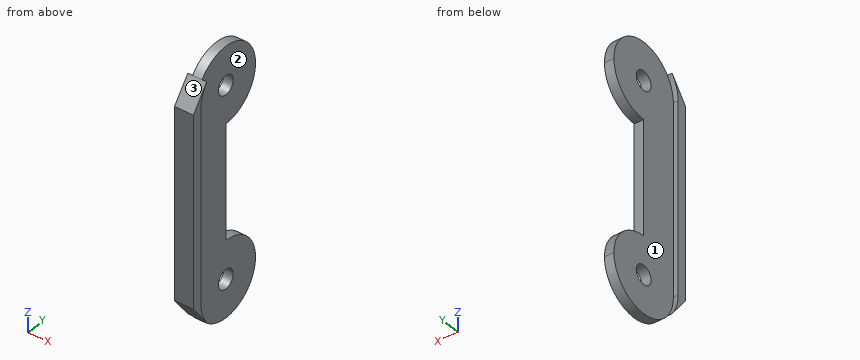
```python
from build123d import *

# Parameters (mm, degrees)
F1_DEPTH = 2.5
F0_R     = 2.5
F2_DEPTH = 1.25


with BuildPart() as f1:
    # F0 (on Right) → F1 (new body, symmetric)
    with BuildSketch(Plane.YZ):
        with BuildLine():
            ThreePointArc((-10, 25), (-9.486833, 28.162278), (-8, 31))
            Line((-8, 31), (-12.5, 25))
            Line((-12.5, 25), (-12.5, -25))
            Line((-12.5, -25), (-8, -31))
            ThreePointArc((-8, -31), (-9.486833, -28.162278), (-10, -25))
            Line((-10, -25), (-10, 25))
        make_face()
    extrude(amount=F1_DEPTH, both=True)

    # F0 (on Right) → F2 (join, symmetric)
    with BuildSketch(Plane.YZ):
        with BuildLine():
            ThreePointArc((0, 15), (7.071068, 17.928932), (10, 25))
            ThreePointArc((10, 25), (3.162278, 34.486833), (-8, 31))
            ThreePointArc((-8, 31), (-9.486833, 28.162278), (-10, 25))
            ThreePointArc((-10, 25), (-7.071068, 17.928932), (0, 15))
        make_face()
        with Locations((0, 25)):
            Circle(F0_R, mode=Mode.SUBTRACT)
        with BuildLine():
            Line((0, -15), (0, 15))
            ThreePointArc((0, 15), (-7.071068, 17.928932), (-10, 25))
            Line((-10, 25), (-10, -25))
            ThreePointArc((-10, -25), (-7.071068, -17.928932), (0, -15))
        make_face()
        with BuildLine():
            ThreePointArc((10, -25), (7.071068, -17.928932), (0, -15))
            ThreePointArc((0, -15), (-7.071068, -17.928932), (-10, -25))
            ThreePointArc((-10, -25), (-9.486833, -28.162278), (-8, -31))
            ThreePointArc((-8, -31), (3.162278, -34.486833), (10, -25))
        make_face()
        with Locations((0, -25)):
            Circle(F0_R, mode=Mode.SUBTRACT)
    extrude(amount=F2_DEPTH, both=True)


solid = f1.part
```
Could you check a few things on this model? Use its own coordinates, in mm. Face numbers are marked on the shaded views. A direction names the side the tool comes from. Coordinates: 2 decimals unless noted, no trailing zeros. Write each loop counter-clockwise with the first axis right and the second up, starting at its lowest first coordinate (ties: lowest second). Pieces come first, ordered by that corner, then holes. Notation, with made-up numbers: (20, 37) -> (36, 37) arc R26 ccw to (36, 65) -> close; hole circle Ø5 at (61.5, 56). An arc over 180 degrees is marked (long way). One line per question, with ' | ' between items. Start each with the question number.
1. If we section it at A-A (y = 8): Please give me the cut outline in (x, z), and give its area (3 significant figures).
2. Will these pins go through, and if not, where does the flat tip stop? P1, Ø1.4, axis at x = 1.5, z = -6, coming from the +Y side; P2, Ø8, axis at y = 0, z = -25, coming from the +X side; P3, Ø2, axis at x = -1, y = 5, coming from the -Z side.
3. If we section it at B-B (x = 0.05): Please give me the cut outline in (y, z).
4. For the marked faces 1, 2 and 3, which set-ups out of +Z, -Z, +X, -X, +Y, -Y let a thin tool reach every point of the face, with its end or its side?
5. If we section it at C-C (z = -13): Please give me the cut outline in (x, y), and give its area (3 significant figures).
6. If we section it at D-D (z = 26): Please give me the cut outline in (x, y).
7. Please list where these lines run through material, in increasing order: line 1 along X through (y, z) = (-5, -5.5); line 2 along Y through (x, z) = (0.1, 6); line 3 along Z through (x, y) = (0.45, 5.5).
Return value:
1) outline: (-1.25, -31) -> (1.25, -31) -> (1.25, -19) -> (-1.25, -19) -> close; (-1.25, 19) -> (1.25, 19) -> (1.25, 31) -> (-1.25, 31) -> close | area: 60.0 mm²
2) P1: stops at y = 0 | P2: stops at x = 1.25 | P3: stops at z = -34.17
3) outline: (-12.5, -25) -> (-8, -31) arc R10 ccw (long way) to (0, -15) -> (0, 15) arc R10 ccw (long way) to (-8, 31) -> (-12.5, 25) -> close; hole circle Ø5 at (0, -25); hole circle Ø5 at (0, 25)
4) face 1: -X, +Y | face 2: +X, +Y | face 3: +Z, +X, -X, -Y
5) outline: (-2.5, -12.5) -> (2.5, -12.5) -> (2.5, -10) -> (1.25, -10) -> (1.25, 0) -> (-1.25, 0) -> (-1.25, -10) -> (-2.5, -10) -> close | area: 37.5 mm²
6) outline: (-2.5, -11.75) -> (2.5, -11.75) -> (2.5, -9.95) -> (1.25, -9.95) -> (1.25, -2.29) -> (-1.25, -2.29) -> (-1.25, -9.95) -> (-2.5, -9.95) -> close; (-1.25, 2.29) -> (1.25, 2.29) -> (1.25, 9.95) -> (-1.25, 9.95) -> close
7) line 1: x = -1.25 to 1.25 | line 2: y = -12.5 to 0 | line 3: z = -33.35 to -16.65, 16.65 to 33.35
